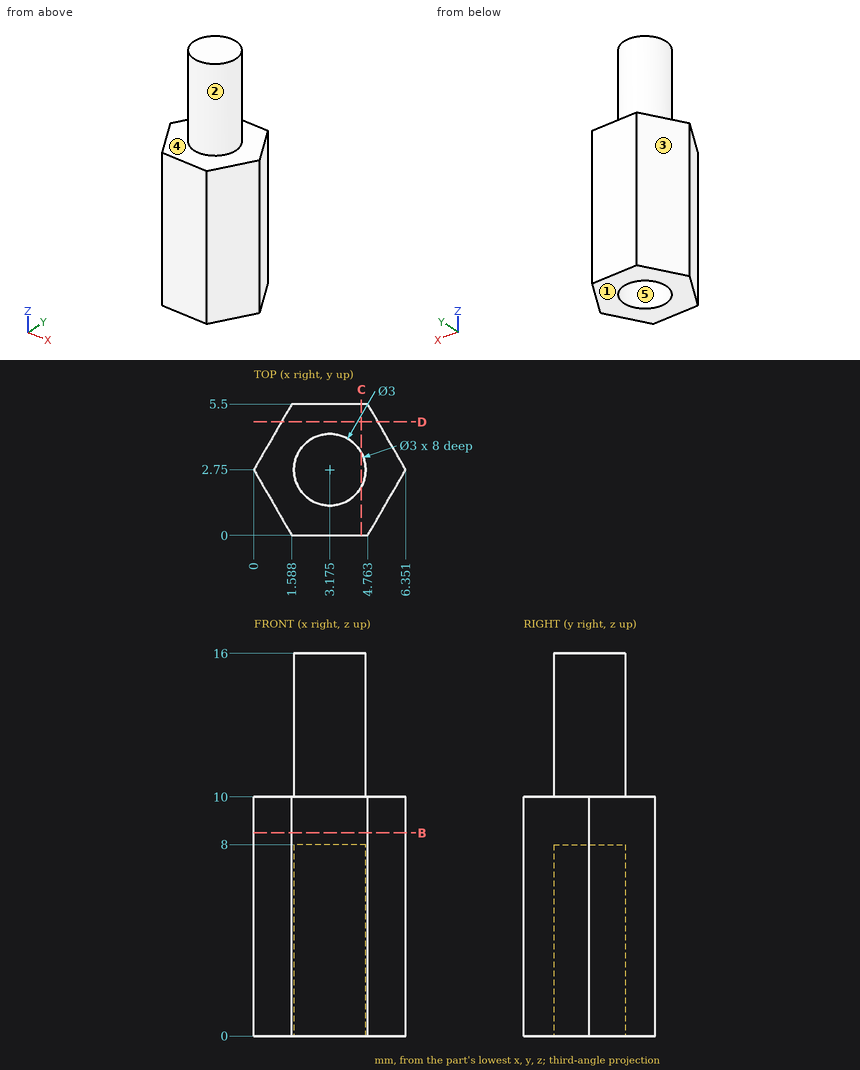
Source: three-view drawing plus pictorial views. Frame: mm from the lowest corner of the part. A direction names the side the tool comes from. Round coordinates to 2 decimals unless told otherwise and drop trailing zeros. Loops run counter-clockwise (first coordinate to the right, second up) from the corner with the lowest first, then second, coordinate; pieces in that order, holes last. Notation, with made-up numbers: M 89,58.5 L 136,58.5 A15 cw 136,80.5 Z; hole C 40.25,49 d7. An arc over 180 degrees is marked long. Put each result on its own line as item: value. Start each with the question number.
(1) Section query B-B (z = 8.5). Return loops of the section in (x, y), then the cut area to 3 significant figures.
(2) Draft query along X for the marked faces 3, 4 and 5. Return one class per face: +X half, -X half, draft (parallel to the pull), parting line (faces both ways), or undercut.
(3) Set-up query: the marked faces 1 and 2. Return all of +Z, -Z, +X, -X, +Y, -Y with unobstructed straight access to the full face (end or side cutting, diameter ignored); none if empty.
(4) Material intervals for line 1 along Z through (x, y) = (1.75, 3.75); line 2 along X through (y, z) = (2.6, 1.5) (1 decimal); line 3 along Z through (x, y) = (3, 1.85), sorted ascending. Write a range as [from, to].
(5) Section query C-C (x = 4.5). Return loops of the section in (y, z).
(6) Section query D-D (y = 4.75). Return loops of the section in (x, z) (1 decimal).
(7) Contact query for flat-ended pins moving along their axis: pin 1 Ø1 at (y, z) = (2, 7.5) entering from +X; pin 2 Ø1.5 at (y, z) = (1, 13.5) entering from -X; pin 3 Ø2 at (y, z) = (2.5, 14) entering from +X (1 decimal). Output: stop coordinate, or through.
Findings below:
1. outline: M 0,2.75 L 1.59,0 L 4.76,0 L 6.35,2.75 L 4.76,5.5 L 1.59,5.5 Z
1. area: 26.2 mm2
2. face 3: -X half
2. face 4: draft
2. face 5: undercut
3. face 1: -Z, +X, -X, +Y, -Y
3. face 2: +Z
4. line 1: z = [0, 10]
4. line 2: x = [0.1, 1.7], [4.7, 6.3]
4. line 3: z = [8, 16]
5. outline: M 0,0 L 2.05,0 L 2.05,8 L 3.45,8 L 3.45,0 L 5.5,0 L 5.5,10 L 3.45,10 L 3.45,16 L 2.05,16 L 2.05,10 L 0,10 Z
6. outline: M 1.2,0 L 5.2,0 L 5.2,10 L 1.2,10 Z
7. pin 1: stops at x = 6.21
7. pin 2: stops at x = 2.06
7. pin 3: stops at x = 4.7
